```python
from build123d import *

# Parameters (mm, degrees)
SKETCH1_W           = 80
SKETCH1_H           = 72.3
BOSS_EXTRUDE1_DEPTH = 6
SKETCH2_W           = 80
SKETCH2_H           = 72.3
SKETCH2_R           = 29.705
CUT_EXTRUDE1_DEPTH  = 3
CUT_EXTRUDE3_DEPTH  = 7
SKETCH5_R           = 2
CUT_EXTRUDE4_DEPTH  = 7
SKETCH6_R           = 2
CUT_EXTRUDE5_DEPTH  = 7
SKETCH8_W           = 6.225749038
SKETCH8_H           = 72.3
BOSS_EXTRUDE2_DEPTH = 15.5


with BuildPart() as part:
    # Sketch1 → Boss-Extrude1 (new body)
    with BuildSketch(Plane(origin=(0, 0, 0), x_dir=(1, 0, 0), z_dir=(0, 1, 0))):
        with Locations((1.546657586, 37.660128709)):
            Rectangle(SKETCH1_W, SKETCH1_H)
    extrude(amount=BOSS_EXTRUDE1_DEPTH)

    # Sketch2 → Cut-Extrude1 (cut)
    with BuildSketch(Plane(origin=(0, 6, 0), x_dir=(-1, 0, 0), z_dir=(0, 1, 0))):
        with Locations((-1.546657586, -37.660128709)):
            Rectangle(SKETCH2_W, SKETCH2_H)
        with Locations((-1.546657586, -37.660128709)):
            Circle(SKETCH2_R, mode=Mode.SUBTRACT)
    extrude(amount=-CUT_EXTRUDE1_DEPTH, mode=Mode.SUBTRACT)

    # Sketch3 → Cut-Extrude3 (cut, through all)
    with BuildSketch(Plane(origin=(0, 6, 0), x_dir=(-1, 0, 0), z_dir=(0, 1, 0))):
        with BuildLine():
            ThreePointArc((-16.671348492, -51.125128709), (-1.546657586, -57.910128709), (13.57803332, -51.125128709))
            Line((13.57803332, -51.125128709), (13.57803332, -45.660128709))
            Line((13.57803332, -45.660128709), (17.056097586, -45.660128709))
            ThreePointArc((17.056097586, -45.660128709), (18.703342414, -37.660128709), (17.056097586, -29.660128709))
            Line((17.056097586, -29.660128709), (13.57803332, -29.660128709))
            Line((13.57803332, -29.660128709), (13.57803332, -24.195128709))
            ThreePointArc((13.57803332, -24.195128709), (-1.546657586, -17.410128709), (-16.671348492, -24.195128709))
            Line((-16.671348492, -24.195128709), (-16.671348492, -29.660128709))
            Line((-16.671348492, -29.660128709), (-20.149412759, -29.660128709))
            Line((-20.149412759, -29.660128709), (-20.149412759, -32.660128709))
            Line((-20.149412759, -32.660128709), (-16.671348492, -32.660128709))
            Line((-16.671348492, -32.660128709), (-16.671348492, -42.660128709))
            Line((-16.671348492, -42.660128709), (-20.149412759, -42.660128709))
            Line((-20.149412759, -42.660128709), (-20.149412759, -45.660128709))
            Line((-20.149412759, -45.660128709), (-16.671348492, -45.660128709))
            Line((-16.671348492, -45.660128709), (-16.671348492, -51.125128709))
        make_face()
    extrude(amount=-CUT_EXTRUDE3_DEPTH, mode=Mode.SUBTRACT)

    # Sketch5 → Cut-Extrude4 (cut, through all)
    with BuildSketch(Plane(origin=(0, 6, 0), x_dir=(-1, 0, 0), z_dir=(0, 1, 0))):
        with Locations((-1.546657586, -12.410128709)):
            Circle(SKETCH5_R)
        with Locations((-1.546657586, -62.910128709)):
            Circle(SKETCH5_R)
    extrude(amount=-CUT_EXTRUDE4_DEPTH, mode=Mode.SUBTRACT)

    # Sketch6 → Cut-Extrude5 (cut, through all)
    with BuildSketch(Plane(origin=(0, 6, 0), x_dir=(1, 0, 0), z_dir=(0, 1, 0))):
        with Locations((-7.953342414, 60.376565813)):
            Circle(SKETCH6_R)
        with Locations((11.046657586, 60.376565813)):
            Circle(SKETCH6_R)
        with Locations((11.046657586, 14.026565813)):
            Circle(SKETCH6_R)
        with Locations((-7.953342414, 14.026565813)):
            Circle(SKETCH6_R)
    extrude(amount=-CUT_EXTRUDE5_DEPTH, mode=Mode.SUBTRACT)

    # Sketch8 → Boss-Extrude2 (add)
    with BuildSketch(Plane(origin=(0, 3, 0), x_dir=(1, 0, 0), z_dir=(0, 1, 0))):
        with Locations((-35.340467895, 37.660128709)):
            Rectangle(SKETCH8_W, SKETCH8_H)
    extrude(amount=BOSS_EXTRUDE2_DEPTH)


solid = part.part
```
Geometry: final body of the model. Coordinates: model frame, mm. A direction names the side the tool comes from. Coordinates: 2 decimals unless noted, no trailing zeros. Loops run counter-clockwise (first coordinate to the right, second up) from the corner with the lowest first, then second, coordinate; pieces in that order, holes last. Notation, with made-up numbers: (-1.5, 59.25) -> (45.5, 59.25) arc R31 cw to (45.5, 90.25) -> close; hole circle Ø8 at (21.25, 4.5). An arc over 180 degrees is marked (long way). Use a Markdown table: item, result. Add a question column.
(1) Section query C-C, the plane x = -20. Return loops of the section in (y, z).
(2) Section query A-A, the plane z = -52.5. Return loops of the section in (x, y), plus the area to 3 significant figures.
(3) Line query: line 1 along Z through (x, y) = (-8, 5.25); line 2 along X through (y, z) = (4, -19.5); line 3 along X through (y, z) = (4.75, -15.5). Output: solid intervals per line, ascending.
(4) Access query for faces 1 (the flat face through (-38.453, 9, -37)), 2 (the flat face through (18, 3, -29.66)). Directions: +Z, -Z, +X, -X, +Y, -Y. A direction counts if a zero-diameter tool reaches every point of the face in a straight line with its end or side. Return the directions, or none.
(5) Pin query (flat end, axial travel): pin 1 Ø6 at (x, z) = (-24.5, -11) entering from -Y; pin 2 Ø4 at (x, y) = (13, 7) entering from -Z; pin 3 Ø2 at (x, z) = (-21.5, -29.5) entering from +Y; pin 4 Ø3 at (x, z) = (1.55, -62.91) entering from +Y. Return the tip coordinate at first contact, or that it passes through.
(6) Section query D-D, the plane z = -9.5. Return loops of the section in (x, y).
(7) Section query B-B, the plane x = -5. Return loops of the section in (y, z).
(8) Mould query, pull axis Z, two halves, no side actions, for faces 3 (the cylindrical face through (1.31, 3.04, -17.41)), 4 (the flat face through (21, 6, -38)), 5 (the flat face through (-10, 2, -73.81)). Classes: pulls with the +Z half, pulls with the -Z half, needs draft (parallel to the pull), parting line crosses it, or undercut.
Answer:
| question | item | result |
|---|---|---|
| 1 | outline | (0, -73.81) -> (3, -73.81) -> (3, -58.11) -> (6, -58.11) -> (6, -17.21) -> (3, -17.21) -> (3, -1.51) -> (0, -1.51) -> close |
| 2 | outline | (-38.45, 0) -> (-12.23, 0) -> (-12.23, 6) -> (-24.19, 6) -> (-24.19, 3) -> (-32.23, 3) -> (-32.23, 18.5) -> (-38.45, 18.5) -> close; (15.32, 0) -> (41.55, 0) -> (41.55, 3) -> (27.28, 3) -> (27.28, 6) -> (15.32, 6) -> close |
| 2 | area | 326 mm^2 |
| 3 | line 1 | z = -65.79 to -62.38, -58.38 to -55.52, -19.8 to -16.03, -12.03 to -9.53 |
| 3 | line 2 | x = -38.45 to -32.23, -21.96 to -7.41, 10.51 to 25.05 |
| 3 | line 3 | x = -38.45 to -32.23, -18.24 to -9.31, -6.6 to 9.69, 12.4 to 21.33 |
| 4 | face 1 | +Z, -Z, -X, +Y, -Y |
| 4 | face 2 | +Y, -Y |
| 5 | pin 1 | stops at y = 0 |
| 5 | pin 2 | stops at z = -65.73 |
| 5 | pin 3 | stops at y = 6 |
| 5 | pin 4 | passes through |
| 6 | outline | (-38.45, 0) -> (41.55, 0) -> (41.55, 3) -> (11, 3) -> (11, 6) -> (-7.91, 6) -> (-7.91, 3) -> (-32.23, 3) -> (-32.23, 18.5) -> (-38.45, 18.5) -> close |
| 7 | outline | (0, -73.81) -> (3, -73.81) -> (3, -66.63) -> (6, -66.63) -> (6, -56.82) -> (0, -56.82) -> close; (0, -18.5) -> (6, -18.5) -> (6, -8.69) -> (3, -8.69) -> (3, -1.51) -> (0, -1.51) -> close |
| 8 | face 3 | undercut |
| 8 | face 4 | needs draft |
| 8 | face 5 | pulls with the -Z half |
